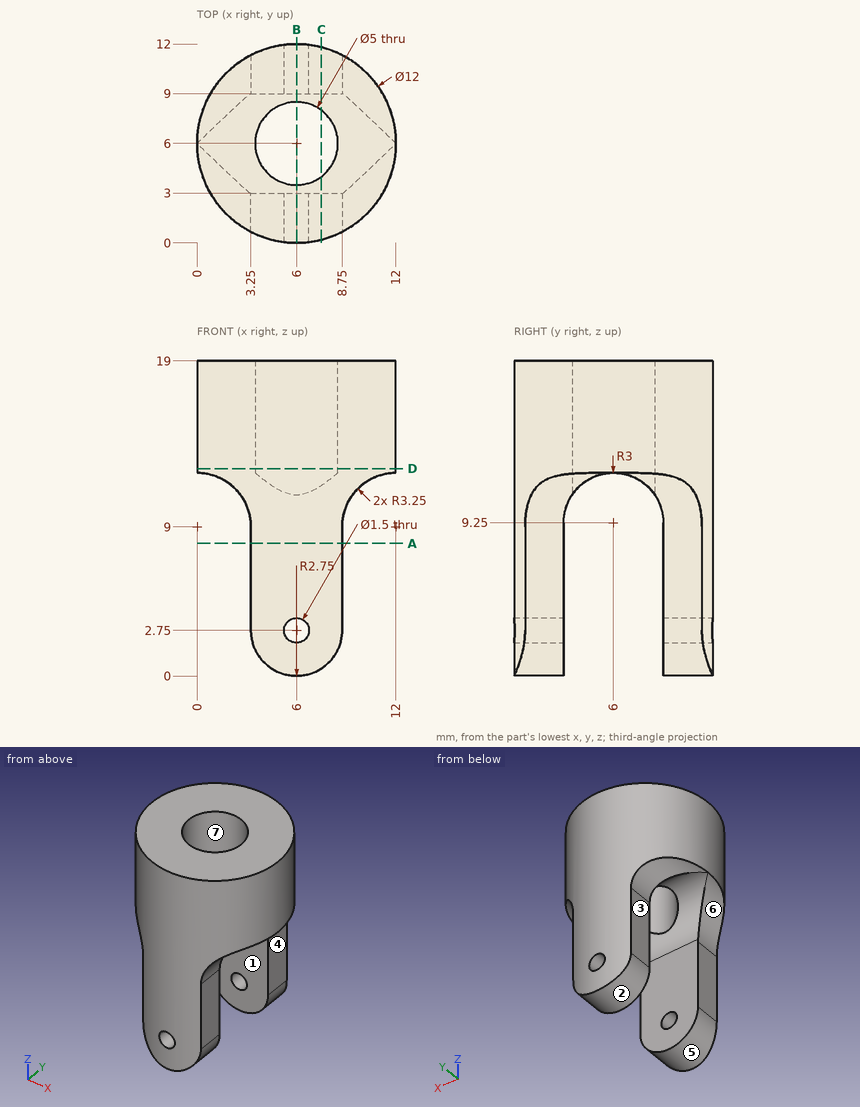
The drawing under review shows one solid part. Ordinate dimensions are in mm from its lowest x, y, z. A direction names the side the tool comes from. Round coordinates to 2 decimals unless told otherwise and drop trailing zeros. Order: outer loops, then holes, each group sorted by start corner. A loop starts at its lowest first (then second) coordinate and runs counter-clockwise, first axis right, second up. Notation, with made-up numbers: (87.5, -10.5) - (146.5, -10.5) arc R25 cw to (146.5, 20.5) - close; hole circle Ø3 at (-20.5, 79). An arc over 180 degrees is marked (long way). Return JSON: item names as keys, results as strings.
Q1. Consider section A-A on z = 8. Write out the cut boundary in (x, y), plus the area to 3 significant figures.
Computed values:
{"outline": "(3.25, 0.67) arc R6 ccw to (8.75, 0.67) - (8.75, 3) - (3.25, 3) - close; (3.25, 9) - (8.75, 9) - (8.75, 11.33) arc R6 ccw to (3.25, 11.33) - close", "area": "30.6 mm2"}
Q2. The part is to be moulded in two halves that separate along X. For the marked faces 5, 6 and 7, say which applies: pulls with the +X half, pulls with the -X half, needs draft (parallel to the pull), parting line crosses it, or undercut.
Computed values:
{"face 5": "parting line crosses it", "face 6": "pulls with the -X half", "face 7": "undercut"}
Q3. Wall thickness on L1, parallel to Y at x = 6, z = 16.75; L2, parallel to Z at x = 6, y = 1.7; L3, parallel to X at y = 9.5, z = 7.25: over which ranges is each line inside the solid? List them lowest first. Write a range as [from, to].
Computed values:
{"L1": "y = [0, 3.5], [8.5, 12]", "L2": "z = [0, 2], [3.5, 19]", "L3": "x = [3.25, 8.75]"}
Q4. Consider section D-D on z = 12.5. Write out the cut boundary in (x, y), plus the area to 3 significant figures.
Computed values:
{"outline": "circle Ø12 at (6, 6); hole circle Ø5 at (6, 6)", "area": "93.5 mm2"}
Q5. Consider section B-B on x = 6. Write out the cut boundary in (y, z), plus the area to 3 significant figures.
Computed values:
{"outline": "(0, 0) - (3, 0) - (3, 2) - (0, 2) - close; (0, 3.5) - (3, 3.5) - (3, 9.25) arc R3 cw to (3.5, 10.91) - (3.5, 19) - (0, 19) - close; (8.5, 10.91) arc R3 cw to (9, 9.25) - (9, 3.5) - (12, 3.5) - (12, 19) - (8.5, 19) - close; (9, 0) - (12, 0) - (12, 2) - (9, 2) - close", "area": "114 mm2"}
Q6. For pin 1 Ø0.7 at (y, z) = (2, 5) entering from -X; pin 2 Ø4 at (x, y) = (3, 5.5) entering from -Z; pin 3 Ø0.7 at (y, z) = (2.5, 5.5) entering from +X, all flat-tipped, find the tip position at first contact; note any pin that passes through.
Computed values:
{"pin 1": "stops at x = 3.25", "pin 2": "stops at z = 10.91", "pin 3": "stops at x = 8.75"}
Q7. Consider section C-C on x = 7.5. Write out the cut boundary in (y, z), plus the area to 3 significant figures.
Computed values:
{"outline": "(0.19, 0.45) - (3, 0.45) - (3, 9.25) arc R3 cw to (4, 11.49) - (4, 19) - (0.19, 19) - close; (8, 11.49) arc R3 cw to (9, 9.25) - (9, 0.45) - (11.81, 0.45) - (11.81, 19) - (8, 19) - close", "area": "121 mm2"}
Q8. Machinability: for the marked faces 1, 2, 3 and 4, which of the approach directions +Z, -Z, +X, -X, +Y, -Y give a long, thin tool a straight path to every point of the face, cutting with its end or side? Answer none if there is none.
Computed values:
{"face 1": "-Z, +X, -X", "face 2": "-Z, +Y, -Y", "face 3": "-Z, -X, +Y, -Y", "face 4": "-Z, +X, +Y, -Y"}
